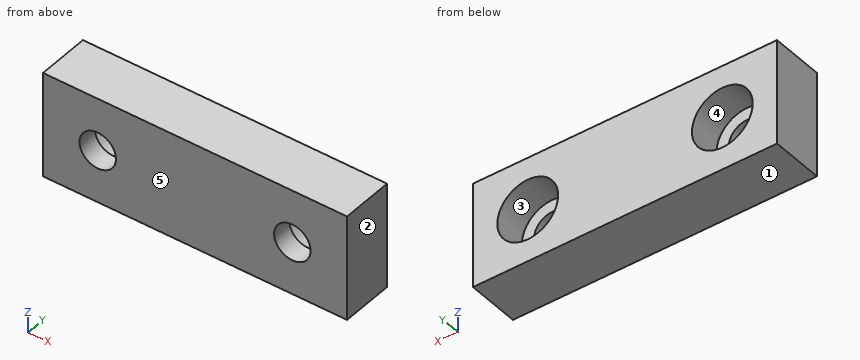
from build123d import *

# Parameters (mm, degrees)
SKETCH1_W                      = 75
SKETCH1_H                      = 26
EXTRUDE1_DEPTH                 = 13
CBORE_FOR_M8_SHCS1_D           = 9
CBORE_FOR_M8_SHCS1_CBORE_D     = 15
CBORE_FOR_M8_SHCS1_CBORE_DEPTH = 8


with BuildPart() as part:
    # Sketch1 → Extrude1 (new body)
    with BuildSketch(Plane(origin=(0, 0, 0), x_dir=(1, 0, 0), z_dir=(0, 1, 0))):
        Rectangle(SKETCH1_W, SKETCH1_H)
    extrude(amount=EXTRUDE1_DEPTH)

    # CBORE for M8 SHCS1 (through all)
    with Locations(Plane(origin=(0, 13, 0), x_dir=(-1, 0, 0), z_dir=(0, 1, 0))):
        with Locations((24, 0)):
            cbore_for_m8_shcs1 = CounterBoreHole(CBORE_FOR_M8_SHCS1_D / 2, CBORE_FOR_M8_SHCS1_CBORE_D / 2, CBORE_FOR_M8_SHCS1_CBORE_DEPTH)

    # Mirror1: CBORE for M8 SHCS1 across plane
    add(cbore_for_m8_shcs1.mirror(Plane(origin=(0, 0, 0), x_dir=(0, 0, 1), z_dir=(1, 0, 0))), mode=Mode.SUBTRACT)


solid = part.part
The model under review builds one solid part; all positions refer to its coordinate system, in mm. Face numbers are marked on the shaded views. A direction names the side the tool comes from. Round coordinates to 2 decimals unless told otherwise and drop trailing zeros. Order: outer loops, then holes, each group sorted by start corner. A loop starts at its lowest first (then second) coordinate and runs counter-clockwise, first axis right, second up. Notation, with made-up numbers: (50.5, 85) -> (91.5, 85) arc R9 ccw to (91.5, 94) -> close; hole circle Ø8 at (39.25, -14). An arc over 180 degrees is marked (long way). Return JSON: item names as keys, results as strings.
1. Insertion check: P1, Ø7.5, axis at x = -23.5, z = -1.5, coming from the +Y side. The pin has a flat end and moves straight along its axis. Give the tip position at first contact, or say it passes through.
Answer block:
{"P1": "stops at y = 5"}
2. Take a section at D-D (z = 6.5). Write out the cut boundary in (x, y), then the cut area to 3 significant figures.
Answer block:
{"outline": "(-37.5, 0) -> (37.5, 0) -> (37.5, 13) -> (27.74, 13) -> (27.74, 5) -> (20.26, 5) -> (20.26, 13) -> (-20.26, 13) -> (-20.26, 5) -> (-27.74, 5) -> (-27.74, 13) -> (-37.5, 13) -> close", "area": "855 mm²"}
3. The part is to be moulded in two halves that separate along X. For the marked faces 1, 2 and 3, say which applies: +X half, -X half, draft (parallel to the pull), parting line (faces both ways), or undercut.
Answer block:
{"face 1": "draft", "face 2": "+X half", "face 3": "undercut"}
4. Take a section at B-B (z = 0). Write out the cut boundary in (x, y), then the cut area to 3 significant figures.
Answer block:
{"outline": "(-37.5, 0) -> (-28.5, 0) -> (-28.5, 5) -> (-31.5, 5) -> (-31.5, 13) -> (-37.5, 13) -> close; (-19.5, 0) -> (19.5, 0) -> (19.5, 5) -> (16.5, 5) -> (16.5, 13) -> (-16.5, 13) -> (-16.5, 5) -> (-19.5, 5) -> close; (28.5, 0) -> (37.5, 0) -> (37.5, 13) -> (31.5, 13) -> (31.5, 5) -> (28.5, 5) -> close", "area": "645 mm²"}
5. For L1, parallel to Z at x = -24, y = 1.85; L2, parallel to X at y = 4.25, z = -1; L3, parallel to X at y = 3.5, z = 3.75, list the stretches that pass through material, from the lowest coordinate up. Write a range as [from, to].
Answer block:
{"L1": "z = [-13, -4.5], [4.5, 13]", "L2": "x = [-37.5, -28.39], [-19.61, 19.61], [28.39, 37.5]", "L3": "x = [-37.5, -26.49], [-21.51, 21.51], [26.49, 37.5]"}
6. Take a section at C-C (y = 1.5). Write out the cut boundary in (x, z).
Answer block:
{"outline": "(-37.5, -13) -> (37.5, -13) -> (37.5, 13) -> (-37.5, 13) -> close; hole circle Ø9 at (-24, 0); hole circle Ø9 at (24, 0)"}
7. Take a section at A-A (x = -24). Write out the cut boundary in (y, z).
Answer block:
{"outline": "(0, -13) -> (13, -13) -> (13, -7.5) -> (5, -7.5) -> (5, -4.5) -> (0, -4.5) -> close; (0, 4.5) -> (5, 4.5) -> (5, 7.5) -> (13, 7.5) -> (13, 13) -> (0, 13) -> close"}
8. For the marked faces 4 and 5, list the 3-axis set-ups (+Z, -Z, +X, -X, +Y, -Y) from which the entire face can be reached by the end or side of a thin tool; tool diameter is ignored.
Answer block:
{"face 4": "+Y", "face 5": "+Z, -Z, +X, -X, -Y"}
